```python
from build123d import *

# Parameters (mm, degrees)
BOSS_EXTRUDE1_DEPTH = 6.223


with BuildPart() as part:
    # Sketch1 → Boss-Extrude1 (new body)
    with BuildSketch(Plane.XY):
        with BuildLine():
            Line((0, 15.9385), (0, 0))
            Line((0, 0), (32.995567884, 0))
            ThreePointArc((32.995567884, 0), (36.801773982, 9.188994382), (38.1, 19.05))
            ThreePointArc((38.1, 19.05), (36.801773982, 28.911005618), (32.995567884, 38.1))
            Line((32.995567884, 38.1), (0, 38.1))
            Line((0, 38.1), (0, 22.1615))
            ThreePointArc((0, 22.1615), (2.20016275, 21.25016275), (3.1115, 19.05))
            ThreePointArc((3.1115, 19.05), (2.20016275, 16.84983725), (0, 15.9385))
        make_face()
        with BuildLine():
            Line((32.995567884, 0), (0, 0))
            Line((0, 0), (0, 15.9385))
            ThreePointArc((0, 15.9385), (-3.1115, 19.05), (0, 22.1615))
            Line((0, 22.1615), (0, 38.1))
            Line((0, 38.1), (32.995567884, 38.1))
            ThreePointArc((32.995567884, 38.1), (-38.1, 19.05), (32.995567884, 0))
        make_face()
        with BuildLine():
            ThreePointArc((38.1, 19.05), (36.801773982, 9.188994382), (32.995567884, 0))
            Line((32.995567884, 0), (178.671098782, 0))
            ThreePointArc((178.671098782, 0), (173.566666667, 19.05), (178.671098782, 38.1))
            Line((178.671098782, 38.1), (32.995567884, 38.1))
            ThreePointArc((32.995567884, 38.1), (36.801773982, 28.911005618), (38.1, 19.05))
        make_face()
        with BuildLine():
            ThreePointArc((178.671098782, 38.1), (173.566666667, 19.05), (178.671098782, 0))
            Line((178.671098782, 0), (211.666666667, 0))
            Line((211.666666667, 0), (211.666666667, 15.9385))
            ThreePointArc((211.666666667, 15.9385), (208.555166667, 19.05), (211.666666667, 22.1615))
            Line((211.666666667, 22.1615), (211.666666667, 38.1))
            Line((211.666666667, 38.1), (178.671098782, 38.1))
        make_face()
        with BuildLine():
            Line((211.666666667, 0), (178.671098782, 0))
            ThreePointArc((178.671098782, 0), (221.527672285, -17.751773982), (249.766666667, 19.05))
            ThreePointArc((249.766666667, 19.05), (221.527672285, 55.851773982), (178.671098782, 38.1))
            Line((178.671098782, 38.1), (211.666666667, 38.1))
            Line((211.666666667, 38.1), (211.666666667, 22.1615))
            ThreePointArc((211.666666667, 22.1615), (213.866829416, 21.25016275), (214.778166667, 19.05))
            ThreePointArc((214.778166667, 19.05), (213.866829416, 16.84983725), (211.666666667, 15.9385))
            Line((211.666666667, 15.9385), (211.666666667, 0))
        make_face()
    extrude(amount=BOSS_EXTRUDE1_DEPTH)


solid = part.part
```
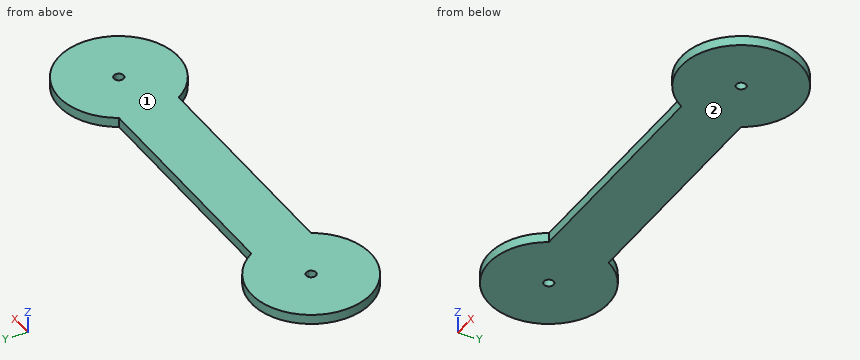
Input: part model. Units: mm. Frame: model coordinates. Face numbers are marked on the shaded views. Round coordinates to 2 decimals unless told otherwise and drop trailing zeros. Loops run counter-clockwise (first coordinate to the right, second up) from the corner with the lowest first, then second, coordinate; pieces in that order, holes last.
1) Pin query (flat end, axial travel): pin 1 (1.9 mm diameter, centred on x = 104, z = 2, fed in from +Y); pin 2 (1.5 mm diameter, centred on y = -10, z = 5.5, fed in from +X); pin 3 (6 mm diameter, centred on x = -0.5, y = -5.5, fed in from -Z); pin 4 (3 mm diameter, centred on x = -7, z = 3, fed in from -Y). Return the tip coordinate at first contact, or that it passes through.
Ans:
pin 1: stops at y = 38.1
pin 2: stops at x = 237.18
pin 3: stops at z = 0
pin 4: stops at y = -18.65
2) Section query C-C on x = 65. Return the cut outline in (y, z).
Ans:
outline: (0, 0) - (38.1, 0) - (38.1, 6.22) - (0, 6.22) - close
3) Material intervals for line 1 (X direction, y = 20, z = 2.5); line 2 (Y direction, x = 138, z = 5); line 3 (X direction, y = -10.5, z = 4.75), sorted ascending.
Ans:
line 1: x = -38.09 to -2.96, 2.96 to 208.7, 214.63 to 249.75
line 2: y = 0 to 38.1
line 3: x = -24.05 to 24.05, 187.62 to 235.72
4) Pull-direction query (Z, two-part tool) for the marked faces 1 and 2; classes: released by +Z, released by -Z, zero draft, split by the parting line, or undercut.
Ans:
face 1: released by +Z
face 2: released by -Z
5) Section query D-D on x = 193.5. Return the cut outline in (y, z).
Ans:
outline: (-14.44, 0) - (52.54, 0) - (52.54, 6.22) - (-14.44, 6.22) - close
6) Section query B-B on y = -12. Return the cut outline in (x, z), plus the area to 3 significant figures.
Ans:
outline: (-22.08, 0) - (22.08, 0) - (22.08, 6.22) - (-22.08, 6.22) - close; (189.59, 0) - (233.75, 0) - (233.75, 6.22) - (189.59, 6.22) - close
area: 550 mm2
7) Section query A-A on z = 5. Return the cut outline in (x, y).
Ans:
outline: (33, 0) - (178.67, 0) arc R38.1 ccw (long way) to (178.67, 38.1) - (33, 38.1) arc R38.1 ccw (long way) to start; hole circle Ø6.22 at (0, 19.05); hole circle Ø6.22 at (211.67, 19.05)
